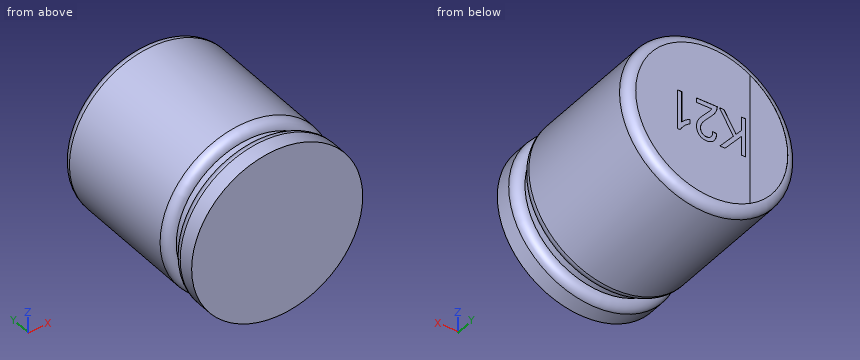
from build123d import *

# Parameters (mm, degrees)
SKETCH1_R           = 9
BOSS_EXTRUDE1_DEPTH = 19.2
FILLET1_R           = 1
CUT_EXTRUDE1_DEPTH  = 0.01
CUT_EXTRUDE2_DEPTH  = 0.01


with BuildPart() as part:
    # Sketch1 → Boss-Extrude1 (new body)
    with BuildSketch(Plane(origin=(0, 0, 0), x_dir=(1, 0, 0), z_dir=(0, 1, 0))):
        Circle(SKETCH1_R)
    extrude(amount=BOSS_EXTRUDE1_DEPTH)

    # Fillet1
    fillet1_edges = [part.edges().sort_by_distance(p)[0] for p in [
        (-9, 19.2, 0),
    ]]
    fillet(fillet1_edges, radius=FILLET1_R)

    # Sketch2 → Cut-Revolve1 (revolve, cut)
    with BuildSketch(Plane.XY):
        with BuildLine():
            Line((-9, 4.7), (-9, 1.7))
            ThreePointArc((-9, 1.7), (-8.707106781, 2.407106781), (-8, 2.7))
            Line((-8, 2.7), (-8, 3.7))
            ThreePointArc((-8, 3.7), (-8.707106781, 3.992893219), (-9, 4.7))
        make_face()
    revolve(axis=Axis((0, -0.75, 0), (0, 1, 0)), mode=Mode.SUBTRACT)

    # Sketch3 → Cut-Extrude1 (cut)
    with BuildSketch(Plane(origin=(0, 19.2, 0), x_dir=(1, 0, 0), z_dir=(0, 1, 0))):
        with BuildLine():
            Line((-4, 6.92820323), (-4, -6.92820323))
            ThreePointArc((-4, -6.92820323), (-8, 0), (-4, 6.92820323))
        make_face()
    extrude(amount=-CUT_EXTRUDE1_DEPTH, mode=Mode.SUBTRACT)

    # Sketch4 → Cut-Extrude2 (cut)
    with BuildSketch(Plane(origin=(0, 19.2, 0), x_dir=(1, 0, 0), z_dir=(0, 1, 0))):
        Polygon((-3.568517869, -2), (-3.568517869, 2.109309896), (-3.141576581, 2.109309896), (-3.141576581, 0.062159775), (-1.398788902, 2.109309896), (-0.855105856, 2.109309896), (-2.27435209, 0.44240436), (-0.793399498, -2), (-1.283714883, -2), (-2.561203268, 0.105521), (-3.141576581, -0.575750547), (-3.141576581, -2), align=None)
        with BuildLine():
            Line((1.608145247, -1.519691051), (1.608145247, -2))
            Line((1.608145247, -2), (-0.579928854, -2))
            add(Edge.make_bspline(
                [(-0.579928854, -2), (-0.580030163, -1.974973894), (-0.580235417, -1.924270595), (-0.573411363, -1.84696894), (-0.559390758, -1.767795767), (-0.541487877, -1.685694894), (-0.516103543, -1.601746123), (-0.485028409, -1.515541552), (-0.448362485, -1.427295796), (-0.405430031, -1.336486232), (-0.355261299, -1.242241802), (-0.29472218, -1.144956808), (-0.22514772, -1.042886175), (-0.146445909, -0.936652158), (-0.057077523, -0.827262261), (0.040304888, -0.713092602), (0.147091103, -0.594380978), (0.223123115, -0.515484132), (0.262279546, -0.474852313)],
                knots=[0, 0, 0, 0, 7.5053e-05, 0.000152058, 0.000232392, 0.000316145, 0.000404002, 0.000495264, 0.000590967, 0.000690561, 0.000796512, 0.000911068, 0.001034111, 0.001167032, 0.001307551, 0.001457781, 0.001617197, 0.001786472, 0.001786472, 0.001786472, 0.001786472], degree=3))
            add(Edge.make_bspline(
                [(0.262279546, -0.474852313), (0.307783709, -0.427786045), (0.395398434, -0.337163605), (0.518707793, -0.20335402), (0.63074673, -0.078979672), (0.729276779, 0.038208492), (0.81604721, 0.146614403), (0.891931027, 0.246083065), (0.953301744, 0.338871858), (1.019564668, 0.4480512), (1.082736953, 0.578027477), (1.138584831, 0.729535393), (1.17466971, 0.875998462), (1.179068277, 0.972558443), (1.181203959, 1.019442194)],
                knots=[0, 0, 0, 0, 0.000196392, 0.000378137, 0.000545859, 0.000698537, 0.000837361, 0.000962441, 0.001073684, 0.001170929, 0.001345461, 0.001506112, 0.00165499, 0.001795499, 0.001795499, 0.001795499, 0.001795499], degree=3))
            add(Edge.make_bspline(
                [(1.181203959, 1.019442194), (1.180906167, 1.045325757), (1.180324549, 1.095879063), (1.17044076, 1.169706759), (1.156345175, 1.239928333), (1.137734826, 1.307051289), (1.111347496, 1.369973118), (1.079731025, 1.429130374), (1.042696817, 1.484790988), (1.00043516, 1.536137563), (0.953830167, 1.582458591), (0.904715044, 1.624072216), (0.851812101, 1.657752353), (0.79729566, 1.687071594), (0.739323506, 1.708320386), (0.679116382, 1.72451746), (0.616117255, 1.733650108), (0.573340408, 1.735033988), (0.551632333, 1.735736269)],
                knots=[0, 0, 0, 0, 7.759e-05, 0.000151542, 0.000223007, 0.000292419, 0.000360091, 0.000427242, 0.000493386, 0.00056033, 0.000626369, 0.000690322, 0.000753001, 0.00081417, 0.000875656, 0.00093775, 0.001000959, 0.001066087, 0.001066087, 0.001066087, 0.001066087], degree=3))
            add(Edge.make_bspline(
                [(0.551632333, 1.735736269), (0.528226771, 1.735245249), (0.48253804, 1.734286754), (0.415943734, 1.722375263), (0.352134158, 1.706440041), (0.291433109, 1.681725902), (0.234284586, 1.650068594), (0.179865337, 1.611963), (0.129240549, 1.566688844), (0.081390427, 1.51520671), (0.0394437, 1.456500761), (0.00093045, 1.392974506), (-0.029397111, 1.321936977), (-0.055184289, 1.245578615), (-0.075379706, 1.163009336), (-0.08887873, 1.074540543), (-0.098778232, 0.980193805), (-0.099334188, 0.9152366), (-0.099619905, 0.881853693)],
                knots=[0, 0, 0, 0, 7.0124e-05, 0.000136886, 0.000202418, 0.000267144, 0.000332829, 0.000398068, 0.000466002, 0.00053623, 0.00060845, 0.0006821, 0.000758639, 0.000839594, 0.000923728, 0.001013247, 0.00110792, 0.001208016, 0.001208016, 0.001208016, 0.001208016], degree=3))
            Line((-0.099619905, 0.881853693), (-0.526561193, 0.935221354))
            add(Edge.make_bspline(
                [(-0.526561193, 0.935221354), (-0.522161355, 0.984764496), (-0.51362547, 1.080880441), (-0.491229682, 1.220023192), (-0.460151497, 1.349122738), (-0.423259749, 1.469467004), (-0.37684568, 1.579562455), (-0.32495328, 1.681412702), (-0.263448356, 1.772803706), (-0.194860218, 1.854865311), (-0.119763265, 1.927670687), (-0.038580752, 1.990514656), (0.048577079, 2.043490936), (0.140714878, 2.088035445), (0.239737182, 2.121299299), (0.343867527, 2.145441457), (0.453952846, 2.159744427), (0.529075899, 2.161685405), (0.567475857, 2.162677557)],
                knots=[0, 0, 0, 0, 0.000149186, 0.000289427, 0.000422308, 0.000547317, 0.00066656, 0.000780315, 0.000889708, 0.000996261, 0.001100641, 0.001202885, 0.001303565, 0.001406135, 0.001509242, 0.001616244, 0.001726397, 0.001841579, 0.001841579, 0.001841579, 0.001841579], degree=3))
            add(Edge.make_bspline(
                [(0.567475857, 2.162677557), (0.608936701, 2.161460519), (0.689667848, 2.159090743), (0.807193372, 2.143475809), (0.916807406, 2.115932118), (1.018999557, 2.077604645), (1.112542526, 2.027147582), (1.198957878, 1.966622956), (1.276803441, 1.894190881), (1.346078887, 1.811773402), (1.407300961, 1.722793837), (1.460721222, 1.629751813), (1.507059009, 1.534189022), (1.543273299, 1.435042114), (1.573516087, 1.33364172), (1.592515267, 1.22845074), (1.605890551, 1.120682885), (1.607389437, 1.047836248), (1.608145247, 1.011103497)],
                knots=[0, 0, 0, 0, 0.000124384, 0.000242196, 0.000354845, 0.000462789, 0.000568739, 0.00067285, 0.000778475, 0.00088674, 0.000995223, 0.001102066, 0.001208364, 0.001313378, 0.001418413, 0.00152537, 0.001633664, 0.001743813, 0.001743813, 0.001743813, 0.001743813], degree=3))
            add(Edge.make_bspline(
                [(1.608145247, 1.011103497), (1.607433131, 0.978008896), (1.606018176, 0.912250864), (1.596813778, 0.814136149), (1.580566309, 0.717340512), (1.559469686, 0.620933232), (1.529533435, 0.526407037), (1.495644001, 0.432260621), (1.454538746, 0.339556084), (1.406012971, 0.24648385), (1.349195592, 0.149750322), (1.281109579, 0.047590004), (1.203017594, -0.062727889), (1.111747658, -0.179237735), (1.011722256, -0.305290035), (0.898522434, -0.437708632), (0.774356786, -0.577661228), (0.686878474, -0.672623554), (0.641690261, -0.721677745)],
                knots=[0, 0, 0, 0, 9.9287e-05, 0.00019728, 0.000295297, 0.000393613, 0.000493053, 0.000592508, 0.000693685, 0.000796994, 0.000907257, 0.001030065, 0.001165193, 0.001312635, 0.001473988, 0.001647918, 0.001835167, 0.002035249, 0.002035249, 0.002035249, 0.002035249], degree=3))
            add(Edge.make_bspline(
                [(0.641690261, -0.721677745), (0.613003238, -0.752199341), (0.558180033, -0.810528561), (0.480543807, -0.894931672), (0.410876198, -0.971712133), (0.347660418, -1.039789018), (0.294021708, -1.101451752), (0.24751759, -1.155071433), (0.209520156, -1.201308971), (0.152573929, -1.273997274), (0.080749983, -1.376414434), (0.031128398, -1.472967089), (0.007115417, -1.519691051)],
                knots=[0, 0, 0, 0, 0.00012566, 0.000240146, 0.000344029, 0.000436694, 0.000518825, 0.000589192, 0.000649623, 0.000698331, 0.000866252, 0.00102371, 0.00102371, 0.00102371, 0.00102371], degree=3))
            Line((0.007115417, -1.519691051), (1.608145247, -1.519691051))
        make_face()
        with BuildLine():
            Line((3.582748703, -2), (3.155807415, -2))
            Line((3.155807415, -2), (3.155807415, 1.25542732))
            add(Edge.make_bspline(
                [(3.155807415, 1.25542732), (3.129587392, 1.225245825), (3.075246421, 1.162694706), (2.980913282, 1.0737383), (2.87578942, 0.982006095), (2.759403349, 0.892993451), (2.640815205, 0.807733741), (2.523687376, 0.732746343), (2.412409759, 0.667501655), (2.337758183, 0.63203815), (2.301924839, 0.615015388)],
                knots=[0, 0, 0, 0, 0.000119871, 0.000248434, 0.000388536, 0.000538317, 0.000687792, 0.000826575, 0.000955448, 0.001074411, 0.001074411, 0.001074411, 0.001074411], degree=3))
            Line((2.301924839, 0.615015388), (2.301924839, 1.095324337))
            add(Edge.make_bspline(
                [(2.301924839, 1.095324337), (2.359511914, 1.12998243), (2.474192959, 1.199001848), (2.634876111, 1.318565767), (2.786671409, 1.447615361), (2.925041729, 1.587502781), (3.048937153, 1.731705768), (3.155279444, 1.875620528), (3.242473386, 2.017717985), (3.285244807, 2.115464643), (3.305903962, 2.162677557)],
                knots=[0, 0, 0, 0, 0.000201529, 0.000401333, 0.000600042, 0.00079875, 0.000990948, 0.001169906, 0.001335222, 0.001489675, 0.001489675, 0.001489675, 0.001489675], degree=3))
            Line((3.305903962, 2.162677557), (3.582748703, 2.162677557))
            Line((3.582748703, 2.162677557), (3.582748703, -2))
        make_face()
    extrude(amount=-CUT_EXTRUDE2_DEPTH, mode=Mode.SUBTRACT)


solid = part.part
Could you check a few things on this model? Use its own coordinates, in mm. Coordinates: 2 decimals unless noted, no trailing zeros. Order: outer loops, then holes, each group sorted by start corner. A loop starts at its lowest first (then second) coordinate and runs counter-clockwise, first axis right, second up. Notation, with made-up numbers: (-26.75, 3) - (-12.75, 3) arc R13 ccw to (-12.75, 17) - close; hole circle Ø3 at (72, 54). An arc over 180 degrees is marked (long way). Answer in a Markdown table with one row per item. Add a question column.
(1) I need wall thicknesses on L1, parallel to Z at x = -5.75, y = 1.25; L2, parallel to Y at x = -5, z = -4.5; L3, parallel to Y at x = 4, z = 7.25. Which ranges of each line are inside material? Lowest first, please.
(2) If we section it at A-A, the plane y = 17.5: Please give me the cut outline in (x, z), then the cut area to 3 significant figures.
(3) Will these pins go through, and if not, where does the flat tip stop? pin 1 (2 mm diameter, centred on x = -6, z = -3, fed in from +Y); pin 2 (1 mm diameter, centred on y = 6, z = -1.5, fed in from +X).
Results are:
| question | item | result |
|---|---|---|
| 1 | L1 | z = -6.92 to 6.92 |
| 1 | L2 | y = 0 to 19.19 |
| 1 | L3 | y = 0 to 2.66, 3.74 to 19.16 |
| 2 | outline | circle Ø18 at (0, 0) |
| 2 | area | 254 mm2 |
| 3 | pin 1 | stops at y = 19.19 |
| 3 | pin 2 | stops at x = 8.94 |
